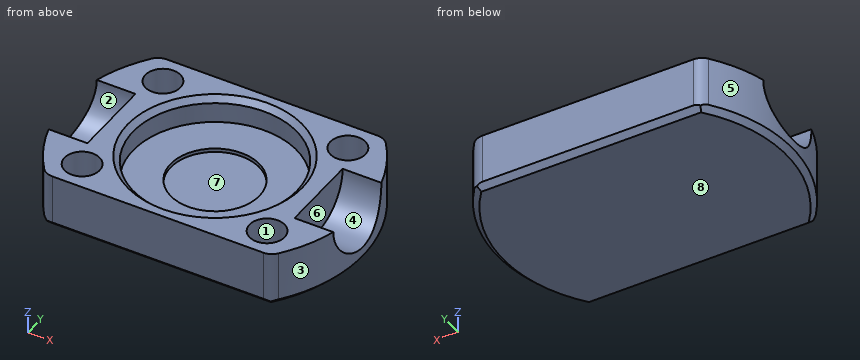
from build123d import *

# Parameters (mm, degrees)
AUFSATZ_LINEAR_AUSTRAGEN1_DEPTH = 7.5
SKIZZE2_R                       = 11.075
SCHNITT_LINEAR_AUSTRAGEN1_DEPTH = 3.5
SKIZZE3_R                       = 5.475
SCHNITT_LINEAR_AUSTRAGEN2_DEPTH = 38.165171868
SKIZZE4_R                       = 2.375
SCHNITT_LINEAR_AUSTRAGEN3_DEPTH = 6
FASE1_SIZE                      = 0.75
VERRUNDUNG1_R                   = 2
SKIZZE5_R                       = 6
SCHNITT_LINEAR_AUSTRAGEN4_DEPTH = 0.5


with BuildPart() as part:
    # Skizze1 → Aufsatz-Linear austragen1 (new body)
    with BuildSketch(Plane.XY):
        with BuildLine():
            Line((-15.198684154, 13), (15.198684154, 13))
            ThreePointArc((15.198684154, 13), (20, 0), (15.198684154, -13))
            Line((15.198684154, -13), (-15.198684154, -13))
            ThreePointArc((-15.198684154, -13), (-20, 0), (-15.198684154, 13))
        make_face()
    extrude(amount=AUFSATZ_LINEAR_AUSTRAGEN1_DEPTH)

    # Skizze2 → Schnitt-Linear austragen1 (cut)
    with BuildSketch(Plane.XY.offset(7.5)):
        Circle(SKIZZE2_R)
    extrude(amount=-SCHNITT_LINEAR_AUSTRAGEN1_DEPTH, mode=Mode.SUBTRACT)

    # Skizze3 → Schnitt-Linear austragen2 (cut, through all)
    with BuildSketch(Plane(origin=(14, 0, 0), x_dir=(0, 0, -1), z_dir=(1, 0, 0))):
        with Locations((-7.5, 0)):
            Circle(SKIZZE3_R)
    schnitt_linear_austragen2 = extrude(amount=SCHNITT_LINEAR_AUSTRAGEN2_DEPTH, mode=Mode.SUBTRACT)

    # Spiegeln1: Schnitt-Linear austragen2 across plane
    add(schnitt_linear_austragen2.mirror(Plane(origin=(0, 0, 0), x_dir=(0, 0, 1), z_dir=(1, 0, 0))), mode=Mode.SUBTRACT)

    # Skizze4 → Schnitt-Linear austragen3 (cut)
    with BuildSketch(Plane.XY.offset(7.5)):
        with Locations((-12.5, 9.2)):
            Circle(SKIZZE4_R)
        with Locations(Location((12.5, 9.2, 0), (0, 0, 180))):
            Circle(SKIZZE4_R)
        with Locations((12.5, -9.2)):
            Circle(SKIZZE4_R)
        with Locations(Location((-12.5, -9.2, 0), (0, 0, 180))):
            Circle(SKIZZE4_R)
    extrude(amount=-SCHNITT_LINEAR_AUSTRAGEN3_DEPTH, mode=Mode.SUBTRACT)

    # Fase1
    fase1_edges = [part.edges().sort_by_distance(p)[0] for p in [
        (-11.075, 0, 7.5),
        (0, 13, 0),
        (20, 0, 0),
        (0, -13, 0),
        (-20, 0, 0),
    ]]
    chamfer(fase1_edges, length=FASE1_SIZE)

    # Verrundung1
    verrundung1_edges = [part.edges().sort_by_distance(p)[0] for p in [
        (-15.198684154, -13, 4.125),
        (15.198684154, -13, 4.125),
        (15.198684154, 13, 4.125),
        (-15.198684154, 13, 4.125),
    ]]
    fillet(verrundung1_edges, radius=VERRUNDUNG1_R)

    # Skizze5 → Schnitt-Linear austragen4 (cut)
    with BuildSketch(Plane.XY.offset(4)):
        Circle(SKIZZE5_R)
    extrude(amount=-SCHNITT_LINEAR_AUSTRAGEN4_DEPTH, mode=Mode.SUBTRACT)


solid = part.part
Design review of the part built by this model. Coordinates are the model's own, in mm. Face numbers are marked on the shaded views. A direction names the side the tool comes from. Give positions to 0.01 mm unless a question says otherwise; leave off trailing zeros. Write each loop counter-clockwise with the first axis right and the second up, starting at its lowest first coordinate (ties: lowest second). Pieces come first, ordered by that corner, then holes. Notation, with made-up numbers: M -40,68.25 L 1,68.25 A26 cw 1,94.25 Z; hole C 63,-12.75 d2. An arc over 180 degrees is marked long. Return JSON: item names as keys, results as strings. Group by question number.
Item 1: Take a section at A-A (x = -12.5). Give the boundary of the cut face in (y, z) (3 decimals), plus the area to 3 significant figures.
Item 2: Tool access review of the marked faces 1, 2, 3, 4 and 5: name each direction out of +Z, -Z, +X, -X, +Y, -Y from which nothing blocks a thin tool from reaching the whole face with its end or side.
Item 3: Take a section at C-C (z = 4.5). Give the boundary of the cut face in (x, y) (3 decimals), plus the area to 3 significant figures.
Item 4: Wall thickness on line 1 along Y through (x, z) = (12.5, 6.35) (3 decimals); line 2 along Y through (x, z) = (0, 3.6); line 3 along Y through (x, z) = (-4, 5): over which ranges is each line inside the solid? List them lowest first.
Item 5: Take a section at D-D (x = 0). Give the boundary of the cut face in (y, z) (3 decimals), plus the area to 3 significant figures.
Item 6: Clearance check with flat-ended pins moving along their axes: pin 1 Ø1.4 at (x, y) = (-12.5, 10) entering from +Z; pin 2 Ø1.6 at (y, z) = (-2.5, 3.5) entering from +X; pin 3 Ø13 at (x, y) = (2.5, -3) entering from +Z. State where each tip first meets the part, or that it passes through.
Item 7: Take a section at B-B (y = 0). Give the boundary of the cut face in (x, z) (3 decimals).
Item 8: The part is to be moulded in two halves that separate along X. For the marked faces 6, 7 and 8, say which applies: pulls with the +X half, pulls with the -X half, needs draft (parallel to the pull), parting line crosses it, or undercut.
Return value:
{
 "1": {"outline": "M -13,0.75 L -12.25,0 L 12.25,0 L 13,0.75 L 13,7.5 L 11.575,7.5 L 11.575,1.5 L 6.825,1.5 L 6.825,7.5 L -6.825,7.5 L -6.825,1.5 L -11.575,1.5 L -11.575,7.5 L -13,7.5 Z", "area": "137 mm2"},
 "2": {"face 1": "+Z", "face 2": "+Z, -X", "face 3": "+Z, -Z, +X", "face 4": "+Z, +X", "face 5": "+Z, -Z, -X"},
 "3": {"outline": "M -19.469,-4.58 A20 ccw -15.831,-12.222 A2 ccw -14.248,-13 L 14.248,-13 A2 ccw 15.831,-12.222 A20 ccw 19.469,-4.58 L 14,-4.58 L 14,4.58 L 19.469,4.58 A20 ccw 15.831,12.222 A2 ccw 14.248,13 L -14.248,13 A2 ccw -15.831,12.222 A20 ccw -19.469,4.58 L -14,4.58 L -14,-4.58 Z; hole C -12.5,-9.2 d4.75; hole C -12.5,9.2 d4.75; hole C 0,0 d22.15; hole C 12.5,-9.2 d4.75; hole C 12.5,9.2 d4.75", "area": "398 mm2"},
 "4": {"line 1": "y = -13 to -11.575, -6.825 to 6.825, 11.575 to 13", "line 2": "y = -13 to -6, 6 to 13", "line 3": "y = -13 to -10.33, 10.33 to 13"},
 "5": {"outline": "M -13,0.75 L -12.25,0 L 12.25,0 L 13,0.75 L 13,7.5 L 11.825,7.5 L 11.075,6.75 L 11.075,4 L 6,4 L 6,3.5 L -6,3.5 L -6,4 L -11.075,4 L -11.075,6.75 L -11.825,7.5 L -13,7.5 Z", "area": "110 mm2"},
 "6": {"pin 1": "stops at z = 1.5", "pin 2": "stops at x = 19.82", "pin 3": "stops at z = 4"},
 "7": {"outline": "M -20,0.75 L -19.25,0 L 19.25,0 L 20,0.75 L 20,2.025 L 14,2.025 L 14,7.5 L 11.825,7.5 L 11.075,6.75 L 11.075,4 L 6,4 L 6,3.5 L -6,3.5 L -6,4 L -11.075,4 L -11.075,6.75 L -11.825,7.5 L -14,7.5 L -14,2.025 L -20,2.025 Z"},
 "8": {"face 6": "pulls with the +X half", "face 7": "undercut", "face 8": "needs draft"}
}
